Model file for the job. Use its own axes, mm. A direction names the side the tool comes from. Give positions to 0.01 mm unless a question says otherwise; leave off trailing zeros. Order: outer loops, then holes, each group sorted by start corner. A loop starts at its lowest first (then second) coordinate and runs counter-clockwise, first axis right, second up. Notation, with made-up numbers: (-18, -23.5) -> (-13, -23.5) arc R25 ccw to (-13, 11.5) -> close; hole circle Ø2 at (3.25, 80.25). An arc over 180 degrees is marked (long way). Use CSV: the item, a comma, the result in double quotes. Start each with the question number.
1. Pull direction Y, two halves, no side cores. Call faces 3 (the cylindrical face through (5.54, 5.44, -2.3)), 4 (the cylindrical face through (-0.54, 2.56, -5.15)), 5 (the cylindrical face through (-11.056, 49.3, 49.787)), 6 (the flat face through (11, 100, -1)): released by +Y, released by -Y, zero draft, split by the parting line, or undercut.
2. Cut at D-D on y = 55.5. List the corners of the cut face in (x, z).
3. Drop flat-ended pins along their axis: pin 1 (2 mm diameter, centred on x = 6, y = 44, fed in from -Z); pin 2 (4 mm diameter, centred on x = 0, y = 5, fed in from +Z); pin 3 (6 mm diameter, centred on x = 0, y = 5, fed in from -Z). Give the stop position or say it passes through.
4. Cut at C-C on x = 44.5. List the corners of the cut face in (y, z), then the cut area to 3 significant figures.
5. Wall check: line 1 (Z direction, x = 0, y = 7.75); line 2 (Y direction, x = 8, z = -5.5); line 3 (X direction, y = 36, z = 0). Give the ranges that are in metal, low to high. Write a range as from..to.
6. Cut at A-A on x = 0. List the corners of the cut face in (y, z), then the cut area to 3 significant figures.
7. 3-axis set-ups, long thin cutter, end or side, ignore diameter. For faces 1 (the flat face through (11, 0, -1)), 2 (the flat face through (-4, 10, 4)): which of +Z, -Z, +X, -X, +Y, -Y reach the whole face in a straight line?
8. Cut at B-B on z = 0. List the corners of the cut face in (x, y), then the cut area to 3 significant figures.
```python
from build123d import *

# Parameters (mm, degrees)
SKETCH1_R               = 51
SKETCH1_R_2             = 50
EXTRUDE_THIN1_DEPTH     = 100
SKETCH1_2_R             = 50
BOSS_EXTRUDE1_DEPTH     = 1
LPATTERN1_COUNT         = 2
LPATTERN1_PITCH         = 99
SKETCH3_R               = 5
CUT_EXTRUDE1_DEPTH      = 101
SKETCH3_2_R             = 6
SKETCH3_2_R_2           = 5
EXTRUDE_THIN2_DEPTH     = 10
SKETCH5_R               = 2.5
CUT_EXTRUDE2_DEPTH      = 20
CUT_EXTRUDE2_DEPTH_BACK = 20


with BuildPart() as part:
    # Sketch1 → Extrude-Thin1 (new body)
    with BuildSketch(Plane(origin=(0, 0, 0), x_dir=(1, 0, 0), z_dir=(0, 1, 0))):
        Circle(SKETCH1_R)
        Circle(SKETCH1_R_2, mode=Mode.SUBTRACT)
    extrude(amount=EXTRUDE_THIN1_DEPTH)

    # Sketch1_2 → Boss-Extrude1 (add)
    with BuildSketch(Plane(origin=(0, 0, 0), x_dir=(1, 0, 0), z_dir=(0, 1, 0))):
        Circle(SKETCH1_2_R)
    boss_extrude1 = extrude(amount=BOSS_EXTRUDE1_DEPTH)

    # LPattern1: Boss-Extrude1 ×2
    with Locations(*[(0, i * LPATTERN1_PITCH, 0) for i in range(1, LPATTERN1_COUNT)]):
        add(boss_extrude1)

    # Sketch3 → Cut-Extrude1 (cut, through all)
    with BuildSketch(Plane.XZ):
        Circle(SKETCH3_R)
    extrude(amount=-CUT_EXTRUDE1_DEPTH, mode=Mode.SUBTRACT)

    # Sketch3_2 → Extrude-Thin2 (add)
    with BuildSketch(Plane.XZ):
        Circle(SKETCH3_2_R)
        Circle(SKETCH3_2_R_2, mode=Mode.SUBTRACT)
    extrude(amount=-EXTRUDE_THIN2_DEPTH)

    # Sketch5 → Cut-Extrude2 (cut, two sides)
    with BuildSketch(Plane.XY) as cut_extrude2_sk:
        with Locations((0, 5)):
            Circle(SKETCH5_R)
    extrude(amount=CUT_EXTRUDE2_DEPTH, mode=Mode.SUBTRACT)
    extrude(cut_extrude2_sk.sketch, amount=-CUT_EXTRUDE2_DEPTH_BACK, mode=Mode.SUBTRACT)


solid = part.part
```
Verdict:
1,face 3,"undercut"
1,face 4,"undercut"
1,face 5,"zero draft"
1,face 6,"released by +Y"
2,outline,"circle Ø102 at (0, 0); hole circle Ø100 at (0, 0)"
3,pin 1,"z = -50.75"
3,pin 2,"z = 51"
3,pin 3,"z = -51"
4,outline,"(0, -24.91) -> (100, -24.91) -> (100, 24.91) -> (0, 24.91) -> close; hole (1, -22.8) -> (99, -22.8) -> (99, 22.8) -> (1, 22.8) -> close"
4,area,"515 mm^2"
5,line 1,"-51..-50, -6..-5, 5..6, 50..51"
5,line 2,"0..1, 99..100"
5,line 3,"-51..-50, 50..51"
6,outline,"(0, -51) -> (100, -51) -> (100, -5) -> (99, -5) -> (99, -50) -> (1, -50) -> (1, -6) -> (2.5, -6) -> (2.5, -5) -> (0, -5) -> close; (0, 5) -> (2.5, 5) -> (2.5, 6) -> (1, 6) -> (1, 50) -> (99, 50) -> (99, 5) -> (100, 5) -> (100, 51) -> (0, 51) -> close; (7.5, -6) -> (10, -6) -> (10, -5) -> (7.5, -5) -> close; (7.5, 5) -> (10, 5) -> (10, 6) -> (7.5, 6) -> close"
6,area,"388 mm^2"
7,face 1,"+Z, -Z, +X, -X, -Y"
7,face 2,"none"
8,outline,"(-51, 0) -> (-5, 0) -> (-5, 10) -> (-6, 10) -> (-6, 1) -> (-50, 1) -> (-50, 99) -> (-5, 99) -> (-5, 100) -> (-51, 100) -> close; (5, 0) -> (51, 0) -> (51, 100) -> (5, 100) -> (5, 99) -> (50, 99) -> (50, 1) -> (6, 1) -> (6, 10) -> (5, 10) -> close"
8,area,"398 mm^2"
